Source: CAD feature listing. Evaluate the final solid. Frame: model axes, mm. Give positions to 0.01 mm unless a question says otherwise; leave off trailing zeros. Order: outer loops, then holes, each group sorted by start corner. A loop starts at its lowest first (then second) coordinate and runs counter-clockwise, first axis right, second up.
1) First-contact query: P1, Ø3, axis at x = -11.77, z = -21.83, coming from the +Y side; P2, Ø1.6, axis at y = 1, z = -12, coming from the -X side; P3, Ø1, axis at y = 1.5, z = -25, coming from the +X side; P4, Ø1.6, axis at x = 12.5, y = 1, coming from the -Z side. Flat tips, straight axial feed; report the tip coordinate or a pass-through.
2) Section B-B, the plane y = 1.75. Give the number of separate pieces and of enclosed holes in the cut face, plus the area to 3 significant figures.
3) Material intervals for line 1 (Z direction, x = 53.5, y = 2.75) (3 decimals); line 2 (Z direction, x = 0.5, y = 0.6) (3 decimals); line 3 (X direction, y = 1, z = -3.5), sorted ascending.
4) Section A-A, the plane x = 50. Return loops of the section in (y, z) (3 decimals), plus the area to 3 significant figures.
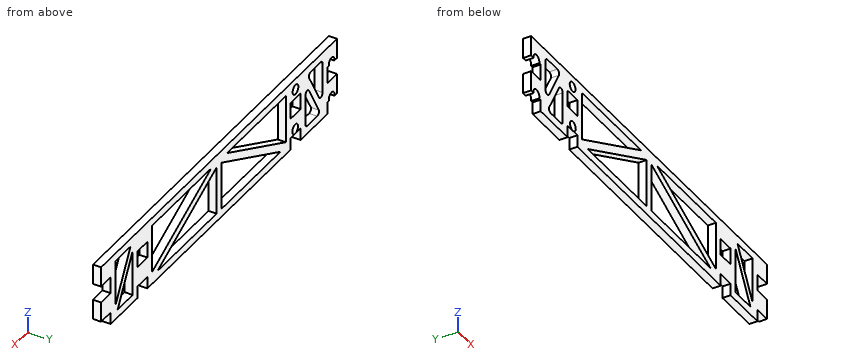
```python
from build123d import *

# Parameters (mm, degrees)
SKETCH1_W                 = 6.5278
SKETCH1_H                 = 6.5278
BOSS_EXTRUDE1_DEPTH       = 3.175
F_6_CLEARANCE_HOLE1_D     = 3.7973
F_6_CLEARANCE_HOLE1_DEPTH = 6.35
F_6_CLEARANCE_HOLE1_TIP   = 1.140824014
FILLET1_R                 = 1.27


with BuildPart() as part:
    # Sketch1 → Boss-Extrude1 (new body)
    with BuildSketch(Plane(origin=(0, 0, 0), x_dir=(1, 0, 0), z_dir=(0, 1, 0))):
        Polygon((110.3249, 27.1653), (15.3289, 27.1653), (15.3289, 22.4028), (8.8011, 22.4028), (8.8011, 27.1653), (-8.9789, 27.1653), (-8.9789, 22.4028), (-15.3289, 22.4028), (-15.3289, 14.4653), (-8.9789, 14.4653), (-8.9789, 7.9375), (-15.3289, 7.9375), (-15.3289, 0), (140.9827, 0), (140.9827, 7.9375), (134.6327, 7.9375), (134.6327, 14.4653), (140.9827, 14.4653), (140.9827, 22.4028), (134.6327, 22.4028), (134.6327, 27.1653), (116.8527, 27.1653), (116.8527, 22.4028), (110.3249, 22.4028), align=None)
        Polygon((-5.8039, 3.175), (-5.8039, 21.351740689), (4.177226675, 3.175), align=None, mode=Mode.SUBTRACT)
        with Locations((12.065, 11.2014)):
            Rectangle(SKETCH1_W, SKETCH1_H, mode=Mode.SUBTRACT)
        Polygon((18.5039, 3.175), (18.5039, 22.224503319), (57.614076125, 3.175), align=None, mode=Mode.SUBTRACT)
        Polygon((107.1499, 3.175), (68.039723875, 3.175), (107.1499, 22.224503319), align=None, mode=Mode.SUBTRACT)
        with Locations((113.5888, 11.2014)):
            Rectangle(SKETCH1_W, SKETCH1_H, mode=Mode.SUBTRACT)
        Polygon((-4.355026675, 23.9903), (5.6261, 23.9903), (5.6261, 5.813559311), align=None, mode=Mode.SUBTRACT)
        Polygon((22.129223875, 23.9903), (61.2394, 23.9903), (61.2394, 4.940796681), align=None, mode=Mode.SUBTRACT)
        Polygon((64.4144, 4.940796681), (64.4144, 23.9903), (103.524576125, 23.9903), align=None, mode=Mode.SUBTRACT)
        Polygon((120.0277, 23.9903), (130.008826675, 23.9903), (120.0277, 5.813559311), align=None, mode=Mode.SUBTRACT)
        Polygon((131.4577, 21.351740689), (131.4577, 3.175), (121.476573325, 3.175), align=None, mode=Mode.SUBTRACT)
    extrude(amount=BOSS_EXTRUDE1_DEPTH)

    # #6 Clearance Hole1
    with Locations(Plane(origin=(11.855385862, 0, -6.482820987), x_dir=(-1, 0, 0), z_dir=(0, -1, 0))):
        with Locations((-0.507300427, 14.014979013), (-0.298514138, -2.158470987), (23.622699573, 1.063018674), (23.622699573, 15.350518674)):
            Hole(F_6_CLEARANCE_HOLE1_D / 2, depth=F_6_CLEARANCE_HOLE1_DEPTH)
            with Locations((0, 0, -(F_6_CLEARANCE_HOLE1_DEPTH + F_6_CLEARANCE_HOLE1_TIP / 2))):  # 118° drill point
                Cone(0, F_6_CLEARANCE_HOLE1_D / 2, F_6_CLEARANCE_HOLE1_TIP, mode=Mode.SUBTRACT)

    # Fillet1
    fillet1_edges = [part.edges().sort_by_distance(p)[0] for p in [
        (-5.8039, 1.5875, -21.351740689),
        (-5.8039, 1.5875, -3.175),
        (4.177226675, 1.5875, -3.175),
        (5.6261, 1.5875, -5.813559311),
        (5.6261, 1.5875, -23.9903),
        (-4.355026675, 1.5875, -23.9903),
    ]]
    fillet(fillet1_edges, radius=FILLET1_R)


solid = part.part
```
From the geometry:
1. P1: passes through
1. P2: stops at x = -8.98
1. P3: stops at x = 134.63
1. P4: stops at z = -22.4
2. separate pieces: 1
2. enclosed holes: 12
2. area: 2,080 mm2
3. line 1: z = -27.165 to -23.99, -8.71 to -5.179, -3.175 to 0
3. line 2: z = -27.165 to -23.99, -15.149 to -9.872, -3.175 to 0
3. line 3: x = -15.33 to -5.38, 2.88 to 10.44, 13.86 to 18.5, 56.95 to 68.71, 107.15 to 121.66, 131.46 to 140.98
4. outline: (0, -27.165) - (3.175, -27.165) - (3.175, -23.99) - (0, -23.99) - close; (0, -10.415) - (3.175, -10.415) - (3.175, -6.884) - (0, -6.884) - close; (0, -3.175) - (3.175, -3.175) - (3.175, 0) - (0, 0) - close
4. area: 31.4 mm2
